```python
from build123d import *

# Parameters (mm, degrees)
SKETCH_2_R               = 16
CUT_EXTRUDE_1_DEPTH      = 1
CUT_EXTRUDE_1_DEPTH_BACK = 51
HOLE_WIZARD_M51_D        = 4.2
HOLE_WIZARD_M51_DEPTH    = 44.001
PATTERN_CIRCULAR_1_COUNT = 6
CHAMFER_1_SIZE           = 0.6


with BuildPart() as part:
    # Эскиз1 → Повернуть1 (revolve)
    with BuildSketch(Plane(origin=(0, 0, 0), x_dir=(1, 0, 0), z_dir=(0, 1, 0))):
        Polygon((0, 0), (-18, 0), (-18, 3), (-28, 3), (-28, 47), (-18, 47), (-18, 50), (0, 50), align=None)
    revolve(axis=Axis((0, 0, -50), (0, 0, 1)))

    # Эскиз2 → Вырез-Вытянуть1 (cut, two sides)
    with BuildSketch(Plane.XY) as cut_extrude_1_sk:
        Circle(SKETCH_2_R)
    extrude(amount=CUT_EXTRUDE_1_DEPTH, mode=Mode.SUBTRACT)
    extrude(cut_extrude_1_sk.sketch, amount=-CUT_EXTRUDE_1_DEPTH_BACK, mode=Mode.SUBTRACT)

    # Сверление под метчик M51
    with Locations(Plane(origin=(23.75, 0, -3), x_dir=(1, 0, 0), z_dir=(0, 0, 1))):
        with Locations((0, 0)):
            hole_wizard_m51 = Hole(HOLE_WIZARD_M51_D / 2, depth=HOLE_WIZARD_M51_DEPTH)

    # Круговой массив1: Сверление под метчик M51 ×6 about axis
    pattern_circular_1_axis = Axis((0, 0, 0), (0, 0, 1))
    for i in range(1, PATTERN_CIRCULAR_1_COUNT):
        add(hole_wizard_m51.rotate(pattern_circular_1_axis, i * 360 / PATTERN_CIRCULAR_1_COUNT), mode=Mode.SUBTRACT)

    # Фаска1
    chamfer_1_edges = [part.edges().sort_by_distance(p)[0] for p in [
        (25.85, 0, -3),
        (25.85, 0, -47),
        (12.925, -22.386756688, -3),
        (12.925, -22.386756688, -47),
        (-12.925, -22.386756688, -3),
        (-12.925, -22.386756688, -47),
        (-25.85, 0, -3),
        (-25.85, 0, -47),
        (-12.925, 22.386756688, -3),
        (-12.925, 22.386756688, -47),
        (12.925, 22.386756688, -3),
        (12.925, 22.386756688, -47),
    ]]
    chamfer(chamfer_1_edges, length=CHAMFER_1_SIZE)


solid = part.part
```
Part model, mm, in its own coordinate system. A direction names the side the tool comes from. Round coordinates to 2 decimals unless told otherwise and drop trailing zeros. Loops run counter-clockwise (first coordinate to the right, second up) from the corner with the lowest first, then second, coordinate; pieces in that order, holes last.
Item 1: Drill centre lines: line 1 (X direction, y = -22, z = -7); line 2 (Y direction, x = 11, z = -11); line 3 (Z direction, x = -12, y = 24.5). Where is each one in solid material? Low to high.
Item 2: 3-axis set-ups, long thin cutter, end or side, ignore diameter. For faces 4 (the face through (-18.3, -0.4, -47)), 5 (the face through (21.747, 0.631, -25.3)), 6 (the face through (18.3, -0.4, -3)): which of +Z, -Z, +X, -X, +Y, -Y reach the whole face in a straight line?
Item 3: Mould opens along Y. For faces 1 (the face through (12, 11, -50)), 2 (the face through (2.343, -17.847, -48.521)), 3 (the face through (13, -22.34, -25.3)) say: +Y half, -Y half, draft (parallel to the pull), parting line (faces both ways), or undercut.
Item 4: Drop flat-ended pins along their axis: P1, Ø2.5, axis at x = -11.87, y = 20.57, coming from the +Z side; P2, Ø5.5, axis at x = 23.75, y = 0, coming from the -Z side; P3, Ø12, axis at x = -13, z = -43, coming from the -Y side; P4, Ø12, axis at y = -18, z = -43, coming from the +X side. Give the stop position or say it passes through.
Item 5: Cut at A-A, the plane y = 0. State how many separate pieces and enclosed holes the cut face has, then the cut area to 3 significant figures.
Item 6: Cut at C-C, the plane y = 9.5. Give the cut face in (x, z), then the cut area to 3 significant figures.
Item 7: Cut at D-D, the plane z = -7.5. Give the cut face in (x, y) (3 decimals).
Item 8: Cut at B-B, the plane x = 0. Give the cut face in (y, z), then the cut area to 3 significant figures.
A:
1. line 1: x = -17.32 to -13.41, -10.34 to 10.34, 13.41 to 17.32
1. line 2: y = -25.75 to -22.48, -18.66 to -11.62, 11.62 to 18.66, 22.48 to 25.75
1. line 3: z = -47 to -3
2. face 4: -Z
2. face 5: +Z, -Z
2. face 6: +Z
3. face 1: draft
3. face 2: parting line
3. face 3: undercut
4. P1: passes through
4. P2: stops at z = -47
4. P3: stops at y = -27.11
4. P4: stops at x = 25.3
5. separate pieces: 4
5. enclosed holes: 0
5. area: 709 mm2
6. outline: (-26.34, -47) - (-15.29, -47) - (-15.29, -50) - (-12.87, -50) - (-12.87, 0) - (-15.29, 0) - (-15.29, -3) - (-26.34, -3) - close; (12.87, -50) - (15.29, -50) - (15.29, -47) - (26.34, -47) - (26.34, -3) - (15.29, -3) - (15.29, 0) - (12.87, 0) - close
6. area: 1,210 mm2
7. outline: circle Ø56 at (0, 0); hole circle Ø4.2 at (-23.75, 0); hole circle Ø32 at (0, 0); hole circle Ø4.2 at (-11.875, -20.568); hole circle Ø4.2 at (-11.875, 20.568); hole circle Ø4.2 at (11.875, -20.568); hole circle Ø4.2 at (11.875, 20.568); hole circle Ø4.2 at (23.75, 0)
8. outline: (-28, -47) - (-18, -47) - (-18, -50) - (-16, -50) - (-16, 0) - (-18, 0) - (-18, -3) - (-28, -3) - close; (16, -50) - (18, -50) - (18, -47) - (28, -47) - (28, -3) - (18, -3) - (18, 0) - (16, 0) - close
8. area: 1,080 mm2
